```python
from build123d import *

# Parameters (mm, degrees)
SKETCH1_W           = 100
SKETCH1_H           = 100
BOSS_EXTRUDE1_DEPTH = 20
SKETCH2_W           = 92
SKETCH2_H           = 92
CUT_EXTRUDE1_DEPTH  = 16
FILLET1_R           = 2
SKETCH3_R           = 2.713966801
CUT_EXTRUDE2_DEPTH  = 16


with BuildPart() as part:
    # Sketch1 → Boss-Extrude1 (new body)
    with BuildSketch(Plane.XY):
        Rectangle(SKETCH1_W, SKETCH1_H)
    extrude(amount=BOSS_EXTRUDE1_DEPTH)

    # Sketch2 → Cut-Extrude1 (cut)
    with BuildSketch(Plane.XY.offset(20)):
        Rectangle(SKETCH2_W, SKETCH2_H)
    extrude(amount=-CUT_EXTRUDE1_DEPTH, mode=Mode.SUBTRACT)

    # Fillet1
    fillet1_edges = [part.edges().sort_by_distance(p)[0] for p in [
        (-46, -46, 12),
        (-46, 46, 12),
        (46, 46, 12),
        (46, -46, 12),
        (-50, 50, 10),
        (50, 50, 10),
        (50, -50, 10),
        (-50, -50, 10),
    ]]
    fillet(fillet1_edges, radius=FILLET1_R)

    # Sketch3 → Cut-Extrude2 (cut)
    with BuildSketch(Plane.XY):
        with Locations((-40, 40)):
            Circle(SKETCH3_R)
        with Locations((40, 40)):
            Circle(SKETCH3_R)
        with Locations((40, -40)):
            Circle(SKETCH3_R)
        with Locations((-40, -40)):
            Circle(SKETCH3_R)
    extrude(amount=CUT_EXTRUDE2_DEPTH, mode=Mode.SUBTRACT)


solid = part.part
```
Work out the finished part from the listing and answer in its coordinate system (mm). A direction names the side the tool comes from. Give positions to 0.01 mm unless a question says otherwise; leave off trailing zeros. Loops run counter-clockwise (first coordinate to the right, second up) from the corner with the lowest first, then second, coordinate; pieces in that order, holes last. Notation, with made-up numbers: (73.5, -15.75) - (105.5, -15.75) arc R30 cw to (105.5, 16.25) - close; hole circle Ø8 at (75, 19). An arc over 180 degrees is marked (long way). One line per question, with ' | ' between items.
(1) The mould has two halves that part along Y. Classify faces 1 (the face through (46, -1, 12)), 2 (the face through (-1, -50, 10)), 3 (the face through (-4, -48, 20)): +Y half, -Y half, draft (parallel to the pull), parting line (faces both ways), or undercut.
Recorded:
face 1: undercut | face 2: -Y half | face 3: draft
(2) The part is cut by section A-A (y = 40). Write down the section's boundary in (x, z).
Recorded:
outline: (-50, 0) - (-42.71, 0) - (-42.71, 4) - (-46, 4) - (-46, 20) - (-50, 20) - close; (-37.29, 0) - (37.29, 0) - (37.29, 4) - (-37.29, 4) - close; (42.71, 0) - (50, 0) - (50, 20) - (46, 20) - (46, 4) - (42.71, 4) - close
(3) The part is cut by section D-D (y = 19). Write down the section's boundary in (x, z), then the cut area to 3 significant figures.
Recorded:
outline: (-50, 0) - (50, 0) - (50, 20) - (46, 20) - (46, 4) - (-46, 4) - (-46, 20) - (-50, 20) - close | area: 528 mm²
(4) The part is cut by section B-B (z = 16). Write down the section's boundary in (x, y), then the cut area to 3 significant figures.
Recorded:
outline: (-50, -48) arc R2 ccw to (-48, -50) - (48, -50) arc R2 ccw to (50, -48) - (50, 48) arc R2 ccw to (48, 50) - (-48, 50) arc R2 ccw to (-50, 48) - close; hole (-46, -44) arc R2 ccw to (-44, -46) - (44, -46) arc R2 ccw to (46, -44) - (46, 44) arc R2 ccw to (44, 46) - (-44, 46) arc R2 ccw to (-46, 44) - close | area: 1,540 mm²
(5) Straight lines are drawn through the part: probe 1 along Y at (x, z) = (40, 1.05); probe 2 along Y at (x, z) = (7, 6.75). For each, find the intervals that lie inside material, in ascending order.
Recorded:
probe 1: y = -50 to -42.71, -37.29 to 37.29, 42.71 to 50 | probe 2: y = -50 to -46, 46 to 50
(6) Each of these flat-tipped pins is pushed along its axis until it touches: pin 1 Ø4.5 at (x, y) = (40, -40) entering from -Z; pin 2 Ø3 at (x, y) = (-35.5, 34.5) entering from -Z; pin 3 Ø6 at (x, y) = (-40, 40) entering from +Z. Where does it stop, or does it pass through?
Recorded:
pin 1: passes through | pin 2: stops at z = 0 | pin 3: stops at z = 4
(7) A tool of negligible diameter and unlimited length cuts with its end or side. For faces 4 (the face through (-1, 50, 10)), 5 (the face through (-46, -1, 12)), from which of +Z, -Z, +X, -X, +Y, -Y can it reach the whole face along a straight path? Write none if from no direction.
Recorded:
face 4: +Z, -Z, +X, -X, +Y | face 5: +Z
